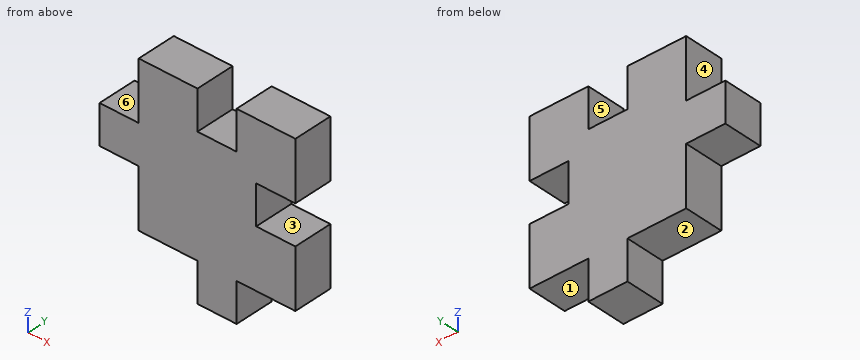
```python
from build123d import *

# Parameters (mm, degrees)
F1_DEPTH = 6.35


with BuildPart() as f1:
    # F0 (on Front) → F1 (new body)
    with BuildSketch(Plane.XZ):
        Polygon((-3.175, 6.35), (-3.175, 12.7), (-12.7, 12.7), (-12.7, 3.175), (-19.05, 3.175), (-19.05, -3.175), (-12.7, -3.175), (-12.7, -12.7), (-3.175, -12.7), (-3.175, -19.05), (3.175, -19.05), (3.175, -12.7), (12.7, -12.7), (12.7, -3.175), (6.35, -3.175), (6.35, 3.175), (12.7, 3.175), (12.7, 12.7), (3.175, 12.7), (3.175, 6.35), (0, 6.35), align=None)
    extrude(amount=F1_DEPTH)


solid = f1.part
```
For this review, take the finished solid that the model builds, in its own axes (mm). Face numbers are marked on the shaded views. A direction names the side the tool comes from. Round coordinates to 2 decimals unless told otherwise and drop trailing zeros. Write each loop counter-clockwise with the first axis right and the second up, starting at its lowest first coordinate (ties: lowest second). Pieces come first, ordered by that corner, then holes.
1) Take a section at B-B on y = -2.5. Give the boundary of the cut face in (x, z) (3 decimals), then the cut area to 3 significant figures.
Answer below:
outline: (-19.05, -3.175) - (-12.7, -3.175) - (-12.7, -12.7) - (-3.175, -12.7) - (-3.175, -19.05) - (3.175, -19.05) - (3.175, -12.7) - (12.7, -12.7) - (12.7, -3.175) - (6.35, -3.175) - (6.35, 3.175) - (12.7, 3.175) - (12.7, 12.7) - (3.175, 12.7) - (3.175, 6.35) - (-3.175, 6.35) - (-3.175, 12.7) - (-12.7, 12.7) - (-12.7, 3.175) - (-19.05, 3.175) - close
area: 645 mm2
2) For line 1 along X through (y, z) = (-2.25, 9.5) (3 decimals); line 2 along Z through (x, y) = (-5, -4.5), list the stretches that pass through material, from the lowest coordinate up.
Answer below:
line 1: x = -12.7 to -3.175, 3.175 to 12.7
line 2: z = -12.7 to 12.7
3) Take a section at C-C on x = -6. Give the boundary of the cut face in (y, z).
Answer below:
outline: (-6.35, -12.7) - (0, -12.7) - (0, 12.7) - (-6.35, 12.7) - close
4) Take a section at D-D on z = -15. Give the boundary of the cut face in (x, y) (3 decimals).
Answer below:
outline: (-3.175, -6.35) - (3.175, -6.35) - (3.175, 0) - (-3.175, 0) - close
5) Insertion check: pin 1 Ø1.9 at (x, y) = (1, -3.5) entering from +Z; pin 2 Ø3 at (y, z) = (-2, 10.5) entering from -X; pin 3 Ø1.9 at (x, y) = (-15, -3.5) entering from -Z (3 decimals). Each pin has a flat end and moves straight along its axis. Give the tip position at first contact, or say it passes through.
Answer below:
pin 1: stops at z = 6.35
pin 2: stops at x = -12.7
pin 3: stops at z = -3.175
6) Take a section at A-A on x = 10. Give the boundary of the cut face in (y, z) (3 decimals).
Answer below:
outline: (-6.35, -12.7) - (0, -12.7) - (0, -3.175) - (-6.35, -3.175) - close; (-6.35, 3.175) - (0, 3.175) - (0, 12.7) - (-6.35, 12.7) - close
7) Machinability: for the marked faces 1, 2 and 3, which of the approach directions +Z, -Z, +X, -X, +Y, -Y give a long, thin tool a straight path to every point of the face, cutting with its end or side? Answer none if there is none.
Answer below:
face 1: -Z, +X, +Y, -Y
face 2: -Z, -X, +Y, -Y
face 3: +X, +Y, -Y
8) Mouldability with a two-part tool opening along X and no side actions: class the marked faces 4, 5 and 6 as +X half, -X half, draft (parallel to the pull), parting line (faces both ways), or undercut.
Answer below:
face 4: -X half
face 5: undercut
face 6: draft
